For this review, use the dimensioned drawing (mm, ordinates from the lowest corner) and the shaded views. Coordinates: 2 decimals unless noted, no trailing zeros. Write each loop counter-clockwise with the first axis right and the second up, starting at its lowest first coordinate (ties: lowest second). Pieces come first, ordered by that corner, then holes.
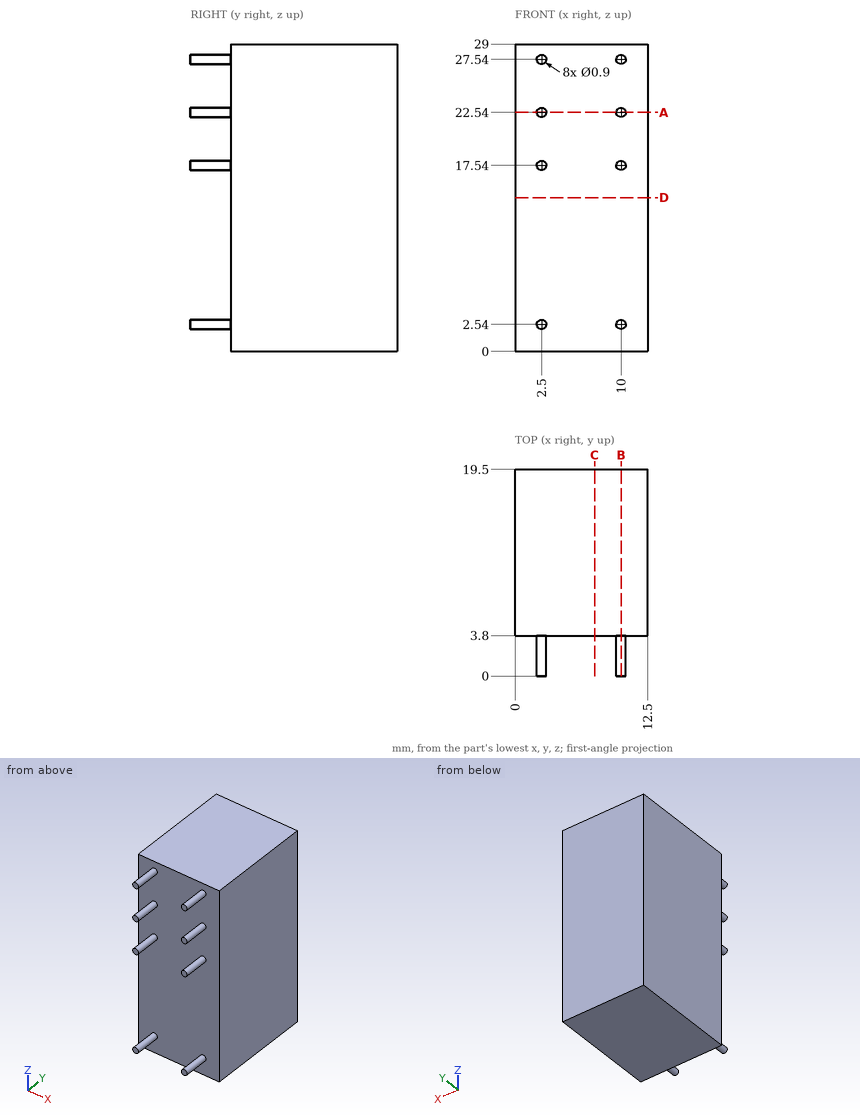
Item 1: Take a section at A-A, the plane z = 22.54. Write out the cut boundary in (x, y), plus the area to 3 significant figures.
Solved:
outline: (0, 3.8) - (2.05, 3.8) - (2.05, 0) - (2.95, 0) - (2.95, 3.8) - (9.55, 3.8) - (9.55, 0) - (10.45, 0) - (10.45, 3.8) - (12.5, 3.8) - (12.5, 19.5) - (0, 19.5) - close
area: 203 mm2
Item 2: To check wall thickness, follow line 1 along Y through (x, z) = (3, 19). State the ranges of the line that lie inside material, in increasing order.
Solved:
line 1: y = 3.8 to 19.5
Item 3: Take a section at C-C, the plane x = 7.5. Write out the cut boundary in (y, z), plus the area to 3 significant figures.
Solved:
outline: (3.8, 0) - (19.5, 0) - (19.5, 29) - (3.8, 29) - close
area: 455 mm2
Item 4: Take a section at D-D, the plane z = 14.5. Write out the cut boundary in (x, y), plus the area to 3 significant figures.
Solved:
outline: (0, 3.8) - (12.5, 3.8) - (12.5, 19.5) - (0, 19.5) - close
area: 196 mm2
Item 5: Take a section at B-B, the plane x = 10. Write out the cut boundary in (y, z).
Solved:
outline: (0, 2.09) - (3.8, 2.09) - (3.8, 0) - (19.5, 0) - (19.5, 29) - (3.8, 29) - (3.8, 27.99) - (0, 27.99) - (0, 27.09) - (3.8, 27.09) - (3.8, 22.99) - (0, 22.99) - (0, 22.09) - (3.8, 22.09) - (3.8, 17.99) - (0, 17.99) - (0, 17.09) - (3.8, 17.09) - (3.8, 2.99) - (0, 2.99) - close
Item 6: For pin 1 (6 mm diameter, centred on x = 3.5, z = 21, fed in from -Y), flat-tipped, find the tip position at first contact; note if it passes through.
Solved:
pin 1: stops at y = 0
